Check sheet for the modelled part. Datum: model origin and axes. Units: mm. A direction names the side the tool comes from. Give positions to 0.01 mm unless a question says otherwise; leave off trailing zeros. Order: outer loops, then holes, each group sorted by start corner. A loop starts at its lowest first (then second) coordinate and runs counter-clockwise, first axis right, second up. Notation, with made-up numbers: (-30.75, -25) -> (-9.75, -25) arc R17 ccw to (-9.75, -2) -> close; hole circle Ø9 at (71.25, -0.5). An arc over 180 degrees is marked (long way). One line per question, with ' | ' between items.
Autodesk Inventor part; units mm, degrees
ref_plane "YZ Plane" through (0, 0, 0) normal (1, 0, 0) x (0, 1, 0)
ref_plane "XZ Plane" through (0, 0, 0) normal (0, 1, 0) x (-1, 0, 0)
ref_plane "XY Plane" through (0, 0, 0) normal (0, 0, 1) x (1, 0, 0)
sketch "Skizze1" plane through (0, 0, 0) normal (1, 0, 0) x (0, 1, 0)
  circle A0 centre (0, 0) radius 12.5
  circle A1 centre (0, 0) radius 16.25
  dimension "d0" = 25
  dimension "d1" = 32.5
extrude "Extrusion1" add sketch "Skizze1" along normal mid plane 0.1
sketch "Skizze2" plane through (0.05, 0, 0) normal (1, 0, 0) x (0, 0, -1)
  circle A0 centre (0, 0) radius 27.5
  dimension "d5" = 55
extrude "Extrusion2" add sketch "Skizze2" along normal blind 22
sketch "Skizze4" plane through (22.05, 0, 0) normal (1, 0, 0) x (0, 0, -1)
  circle A0 centre (0, 0) radius 12.5
  dimension "d8" = 25
extrude "Extrusion3" cut sketch "Skizze4" against normal blind 30
sketch "Skizze5" plane through (0.05, 0, 0) normal (-1, 0, 0) x (0, 0, 1)
  point P0 (0, 0)
  point P1 (0.0333, -22)
  point P2 (19.0692, -10.9712)
  point P3 (19.0359, 11.0288)
  point P4 (-0.0333, 22)
  point P5 (-19.0692, 10.9712)
  point P6 (-19.0359, -11.0288)
  dimension "d18" = 22
  dimension "d21" = 360
hole "Bohrung1" at (0.05, -22, 0.0333) at (0.05, -10.9712, 19.0692) at (0.05, 11.0288, 19.0359) at (0.05, 22, -0.0333) at (0.05, 10.9712, -19.0692) at (0.05, -11.0288, -19.0359) direction (1, 0, 0) diameter 4.917 depth 12.8 tip angle 118
sketch "Skizze6" plane through (22.05, 0, 0) normal (1, 0, 0) x (0, 0, -1)
  line L0 (-16, -4) -> (-9, -4)
  line L1 (-9, -4) -> (-9, 4)
  line L2 (-9, 4) -> (-16, 4)
  line L3 (-16, 4) -> (-16, -4)
  circle A0 centre (0, 0) radius 12.5
  line L4 (-16, -4) -> (-9, 4) construction
  line L5 (-9, -4) -> (-16, 4) construction
  point P0 (-12.5, 0)
  point P1 (-11.8427, -4)
  point P2 (-11.8427, 4)
  dimension "d23" = 7
  dimension "d24" = 8
  dimension "d25" = 9
extrude "Extrusion4" cut sketch "Skizze6" against normal blind 52 contours L3 L2 A0 L0
properties part number "Befestigung bremsscheibe"
Q1. Section check D-D (z = -14.5). Enter the section's corners in (x, y), and give its area (3 significant figures).
Result sheet:
outline: (-0.05, -7.34) -> (0.05, -7.34) -> (0.05, -23.37) -> (22.05, -23.37) -> (22.05, 23.37) -> (0.05, 23.37) -> (0.05, 7.34) -> (-0.05, 7.34) -> close | area: 1,030 mm2
Q2. Section check B-B (z = 7.5). Enter the section's corners in (x, y).
Result sheet:
outline: (-0.05, -14.42) -> (0.05, -14.42) -> (0.05, -26.46) -> (22.05, -26.46) -> (22.05, -10) -> (-0.05, -10) -> close; (-0.05, 10) -> (22.05, 10) -> (22.05, 26.46) -> (0.05, 26.46) -> (0.05, 14.42) -> (-0.05, 14.42) -> close
Q3. Mould release check, pull along Y, two halves, no side actions. Record for faces 1 (the face through (0.05, -12, -12)), 2 (the face through (14.071, -10.669, -18.806)): pulls with the +Y half, pulls with the -Y half, needs draft (parallel to the pull), parting line crosses it, or undercut.
Result sheet:
face 1: needs draft | face 2: undercut
Q4. Access from +Z, -Z, +X, -X, +Y, -Y to the whole of each face (thin tool, end or side, straight path). Record for faces 3 (the face through (11, 0, 16)), 4 (the face through (-0.05, -5, -12)), 5 (the face through (6.54, -10.087, -16.765)).
Result sheet:
face 3: +X, -X | face 4: +Z, -Z, -X, +Y, -Y | face 5: -X
Q5. Depth check by flat-ended pin: pin 1 Ø8 at (x, y) = (18, -15.5) entering from -Z; pin 2 Ø4 at (x, z) = (10.5, -13) entering from +Y; pin 3 Ø6.5 at (y, z) = (-10.97, 19.07) entering from -X. Enter the tip coordinate at first touch or a pass-through.
Result sheet:
pin 1: stops at z = -24.98 | pin 2: stops at y = 25.2 | pin 3: stops at x = 0.05
Q6. Thickness scan on line 1 (Z direction, x = 1.5, y = 0.5); line 2 (Y direction, x = 13, z = 0); line 3 (Y direction, x = 11.75, z = -6.5). Record the ranges inside material, lowest first.
Result sheet:
line 1: z = -27.5 to -12.49, 16 to 27.5 | line 2: y = -27.5 to -24.21, -19.79 to -12.5, 12.5 to 19.79, 24.21 to 27.5 | line 3: y = -26.72 to -10.68, 10.68 to 26.72
Q7. Section check A-A (y = 0). Enter the section's corners in (x, z).
Result sheet:
outline: (-0.05, -16.25) -> (0.05, -16.25) -> (0.05, -27.5) -> (22.05, -27.5) -> (22.05, -12.5) -> (-0.05, -12.5) -> close; (-0.05, 16) -> (22.05, 16) -> (22.05, 27.5) -> (0.05, 27.5) -> (0.05, 16.25) -> (-0.05, 16.25) -> close
Q8. Section check C-C (x = 10.5). Enter the section's corners in (y, z), and give its area (3 significant figures).
Result sheet:
outline: circle Ø55 at (0, 0); hole circle Ø4.92 at (-22, 0.03); hole circle Ø4.92 at (-11.03, -19.04); hole circle Ø4.92 at (-10.97, 19.07); hole (-4, 11.84) arc R12.5 ccw (long way) to (4, 11.84) -> (4, 16) -> (-4, 16) -> close; hole circle Ø4.92 at (10.97, -19.07); hole circle Ø4.92 at (11.03, 19.04); hole circle Ø4.92 at (22, -0.03) | area: 1,740 mm2
